```python
from build123d import *
from build123d.topology import SkipClean

# Parameters (mm, degrees)
EXTRUDE_1_DEPTH     = 10
SKETCH_2_R          = 2.500000000000002
SKETCH_2_R_2        = 2.5
CUT_EXTRUDE_1_DEPTH = 10
EXTRUDE_START       = -27.850000000000005
SKETCH_4_R          = 4.999999999999997
EXTRUDE_2_DEPTH     = 27.850000000000005
EXTRUDE_START_2     = -10
EXTRUDE_3_DEPTH     = 10
FILLET_1_R          = 2
CHAMFER_START       = 4
CHAMFER_1_OUTLINE_W = 8.394855713999998
CHAMFER_1_OUTLINE_H = 10
CHAMFER_1_DEPTH     = 3.536622653
SKETCH_6_R          = 2.500000000000002
CUT_EXTRUDE_2_DEPTH = 8
SKETCH_8_R          = 1.7500000000000036
CUT_EXTRUDE_4_DEPTH = 10.85
SKETCH_9_R          = 2.500000000000002
CUT_EXTRUDE_5_DEPTH = 9
CUT_EXTRUDE_START   = -3
CUT_EXTRUDE_6_DEPTH = 4
FILLET_2_R          = 1
EXTRUDE_START_3     = 4
EXTRUDE_4_DEPTH     = 4
SKETCH_12_R         = 2.5
EXTRUDE_5_DEPTH     = 4


with BuildPart() as part:
    # 草图1 → 凸台-拉伸1 (new body)
    with BuildSketch(Plane.XY):
        with BuildLine():
            Line((0, 5), (50, 5.000000000000001))
            ThreePointArc((50, 5.000000000000001), (55, 0), (50, -4.999999999999997))
            Line((50, -4.999999999999997), (0, -5))
            ThreePointArc((0, -5), (-5, 6.1e-16), (0, 5))
        make_face()
    extrude(amount=EXTRUDE_1_DEPTH)

    # 草图2 → 切除-拉伸1 (cut)
    with BuildSketch(Plane.XY.offset(10)):
        with Locations((50, 0)):
            Circle(SKETCH_2_R)
        Circle(SKETCH_2_R_2)
    extrude(amount=-CUT_EXTRUDE_1_DEPTH, mode=Mode.SUBTRACT)

    # 草图4 → 凸台-拉伸2 (add)
    with SkipClean():  # the faces are left unmerged after this step: merging them gives an invalid solid
        with BuildSketch(Plane.XY.offset(10).offset(EXTRUDE_START)):
            with Locations(Location((50, 0, 0), (0, 0, 270))):
                Circle(SKETCH_4_R)
        extrude(amount=EXTRUDE_2_DEPTH)

    # 草图5 → 凸台-拉伸3 (add)
    with SkipClean():  # the faces are left unmerged after this step: merging them gives an invalid solid
        with BuildSketch(Plane.XY.offset(10).offset(EXTRUDE_START_2)):
            with BuildLine():
                Line((-9.171946933133274, -2.4749524148530857), (-4.827340491122777, -1.3026065341332034))
                ThreePointArc((-4.827340491122777, -1.3026065341332034), (-3.0403097974823012, -3.9694478627805583), (5.411e-14, -5))
                Line((5.411e-14, -5), (1.028e-13, -9.5))
                ThreePointArc((1.028e-13, -9.5), (-5.7765886152163715, -7.541950939283059), (-9.171946933133274, -2.4749524148530857))
            make_face()
        extrude(amount=EXTRUDE_3_DEPTH)

    # 圆角1
    fillet_1_edges = [part.edges().sort_by_distance(p)[0] for p in [
        (1.028e-13, -9.5, 5),
    ]]
    fillet(fillet_1_edges, radius=FILLET_1_R)

    # 倒角1: read off the stored shape, not the designer's step
    # 倒角1 outline → 倒角1 (add)
    with BuildSketch(Plane(origin=(0, 0, 0), x_dir=(0.9076430982816491, 0.41974278569343915, 0), z_dir=(0.41974278569343915, -0.9076430982816494, 0)).offset(CHAMFER_START)):
        with Locations((0.18755170199999993, 5)):
            Rectangle(CHAMFER_1_OUTLINE_W, CHAMFER_1_OUTLINE_H)
    extrude(amount=CHAMFER_1_DEPTH)

    # 草图6 → 切除-拉伸2 (cut)
    with BuildSketch(Plane(origin=(0, 0, -17.850000000000005), x_dir=(-1, 0, 0), z_dir=(0, 0, -1))):
        with Locations((-50, 0)):
            Circle(SKETCH_6_R)
    extrude(amount=-CUT_EXTRUDE_2_DEPTH, mode=Mode.SUBTRACT)

    # 草图8 → 切除-拉伸4 (cut)
    with BuildSketch(Plane(origin=(0, 0, -9.850000000000005), x_dir=(-1, 0, 0), z_dir=(0, 0, -1))):
        with Locations((-50, 0)):
            Circle(SKETCH_8_R)
    extrude(amount=-CUT_EXTRUDE_4_DEPTH, mode=Mode.SUBTRACT)

    # 草图9 → 切除-拉伸5 (cut)
    with BuildSketch(Plane(origin=(0, 0, 1.0000000000000009), x_dir=(-1, 0, 0), z_dir=(0, 0, -1))):
        with Locations((-50, 0)):
            Circle(SKETCH_9_R)
    extrude(amount=-CUT_EXTRUDE_5_DEPTH, mode=Mode.SUBTRACT)

    # 草图10 → 切除-拉伸6 (cut)
    with BuildSketch(Plane(origin=(0, 0, 0), x_dir=(-1, 0, 0), z_dir=(0, 0, -1)).offset(CUT_EXTRUDE_START)):
        with BuildLine():
            Line((3.5355339059327444, -3.535533905932731), (6.717514421272216, -6.717514421272188))
            ThreePointArc((6.717514421272216, -6.717514421272188), (8.223051661510107, -4.757249349375738), (9.171946933133274, -2.474952414853084))
            Line((9.171946933133274, -2.474952414853084), (4.827340491122777, -1.3026065341332023))
            ThreePointArc((4.827340491122777, -1.3026065341332023), (-4.327921927110582, 2.503815447039863), (3.5355339059327444, -3.535533905932731))
        make_face()
    extrude(amount=-CUT_EXTRUDE_6_DEPTH, mode=Mode.SUBTRACT)

    # 圆角2
    fillet_2_edges = [part.edges().sort_by_distance(p)[0] for p in [
        (-3.1e-16, 5, 5),
    ]]
    fillet(fillet_2_edges, radius=FILLET_2_R)

    # 草图11 → 凸台-拉伸4 (add)
    with BuildSketch(Plane(origin=(0, 0, 7), x_dir=(-1, 0, 0), z_dir=(0, 0, -1)).offset(EXTRUDE_START_3)):
        with BuildLine():
            Line((8.197358015291606, -4.801387462925119), (3.5463669464222503, -3.5463669464222334))
            Line((3.5463669464222494, -3.5463669464222356), (6.717514421272216, -6.717514421272188))
            ThreePointArc((6.717514421272217, -6.71751442127219), (7.518725994466674, -5.8067856357998195), (8.197358015291606, -4.801387462925119))
        make_face()
    extrude(amount=-EXTRUDE_4_DEPTH)

    # 草图12 → 凸台-拉伸5 (add)
    with BuildSketch(Plane(origin=(0, 0, 7), x_dir=(-1, 0, 0), z_dir=(0, 0, -1)).offset(EXTRUDE_START_3)):
        with BuildLine():
            Line((3.546366946422246, -3.546366946422232), (8.197358015291606, -4.80138746292512))
            ThreePointArc((8.197358015291606, -4.80138746292512), (8.762206548927544, -3.6706588501155046), (9.171946933133276, -2.474952414853084))
            Line((9.171946933133276, -2.474952414853084), (4.827340491122777, -1.3026065341332018))
            ThreePointArc((4.827340491122777, -1.3026065341332018), (3.9694478627805414, 3.040309797482321), (3.1e-16, 5))
            Line((3.1e-16, 5), (-4.47213595499958, 5))
            ThreePointArc((-4.47213595499958, 5), (-3.5592650258243026, 4.408248290463862), (-3.7267799624996503, 3.333333333333333))
            ThreePointArc((-3.7267799624996503, 3.333333333333333), (-3.4357645511885355, -3.6325641011269494), (3.535533905932743, -3.5355339059327324))
            Line((3.535533905932743, -3.5355339059327324), (3.546366946422246, -3.546366946422232))
        make_face()
        with Locations(Location((0, 0, 0), (0, 0, 180))):
            Circle(SKETCH_12_R, mode=Mode.SUBTRACT)
    extrude(amount=-EXTRUDE_5_DEPTH)


solid = part.part
```
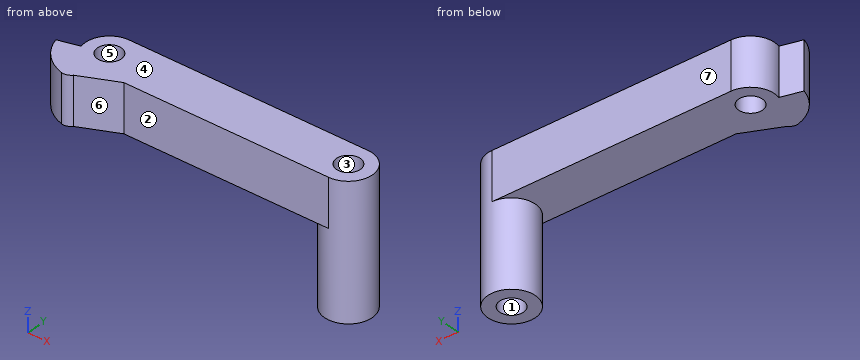
The model under review builds one solid part; all positions refer to its coordinate system, in mm. Face numbers are marked on the shaded views. A direction names the side the tool comes from. Round coordinates to 2 decimals unless told otherwise and drop trailing zeros. Order: outer loops, then holes, each group sorted by start corner. A loop starts at its lowest first (then second) coordinate and runs counter-clockwise, first axis right, second up. Notation, with made-up numbers: (-3.5, 54.25) -> (29.5, 54.25) arc R29 cw to (29.5, 88.25) -> close; hole circle Ø4 at (67.25, -16.75). An arc over 180 degrees is marked (long way). One line per item, written item: value. Start each with the question number.
Q1. Take a section at B-B (z = 2.25). Write out the cut boundary in (x, y).
Q2. Take a section at D-D (x = 22). Write out the cut boundary in (y, z), and give its area (3 significant figures).
Q3. Clearance check with flat-ended pins moving along their axes: pin 1 Ø6 at (y, z) = (-3, -3.5) entering from -X; pin 2 Ø11 at (x, z) = (36.5, 3) entering from -Y; pin 3 Ø4 at (x, y) = (49.5, 1) entering from -Z; pin 4 Ø7 at (x, y) = (10, -4.5) entering from -Z. State where each tip first meets the part, or that it passes through.
Q4. Machinability: for the marked faces 1, 2, 3 and 4, which of the approach directions +Z, -Z, +X, -X, +Y, -Y give a long, thin tool a straight path to every point of the face, cutting with its end or side? Answer none if there is none.
Q5. Wall thickness on line 1 (Y direction, x = 50, z = -15.5); line 2 (X direction, y = 0.25, z = -11); line 3 (Y direction, x = 50, z = -6.5): over which ranges is each line inside the solid? List them lowest first.
Q6. Take a section at C-C (z = -4.5). Write out the cut boundary in (x, y).
Q7. Take a section at A-A (y = 0). Write out the cut boundary in (x, z), and give its area (3 significant figures).
Q8. Mouldability with a two-part tool opening along X and no side actions: class the marked faces 5, 6 and 7 as released by +X, released by -X, zero draft, split by the parting line, or undercut.
Reported:
1. outline: (-9.17, -2.47) arc R9.5 ccw to (-2.53, -9.16) arc R2 ccw to (-0.48, -8.52) -> (7.14, -5) -> (50, -5) arc R5 ccw to (50, 5) -> (0, 5) arc R5 ccw to (-4.83, -1.3) -> close; hole circle Ø5 at (0, 0); hole circle Ø5 at (50, 0)
2. outline: (-5, 0) -> (5, 0) -> (5, 10) -> (-5, 10) -> close
2. area: 100 mm2
3. pin 1: stops at x = 45
3. pin 2: stops at y = -5
3. pin 3: stops at z = -17.85
3. pin 4: stops at z = 0
4. face 1: -Z
4. face 2: +Z, -Z, +X, -Y
4. face 3: +Z
4. face 4: +Z, +X, -X, +Y, -Y
5. line 1: y = -5 to -2.5, 2.5 to 5
5. line 2: x = 45.01 to 47.51, 52.49 to 54.99
5. line 3: y = -5 to -1.75, 1.75 to 5
6. outline: circle Ø10 at (50, 0); hole circle Ø3.5 at (50, 0)
7. outline: (-5, 0) -> (-2.5, 0) -> (-2.5, 10) -> (-5, 10) -> close; (2.5, 0) -> (45, 0) -> (45, -17.85) -> (47.5, -17.85) -> (47.5, -9.85) -> (48.25, -9.85) -> (48.25, 1) -> (47.5, 1) -> (47.5, 10) -> (2.5, 10) -> close; (51.75, -9.85) -> (52.5, -9.85) -> (52.5, -17.85) -> (55, -17.85) -> (55, 10) -> (52.5, 10) -> (52.5, 1) -> (51.75, 1) -> close
7. area: 606 mm2
8. face 5: undercut
8. face 6: released by +X
8. face 7: zero draft
